Design review of the part built by this model. Coordinates are the model's own, in mm. Face numbers are marked on the shaded views. A direction names the side the tool comes from. Round coordinates to 2 decimals unless told otherwise and drop trailing zeros. Loops run counter-clockwise (first coordinate to the right, second up) from the corner with the lowest first, then second, coordinate; pieces in that order, holes last. Notation, with made-up numbers: M -24.5,34.25 L -17.5,34.25 A7 cw -17.5,46.25 Z; hole C -34.75,-6 d4. An arc over 180 degrees is marked long. Use a Markdown table: item, result.
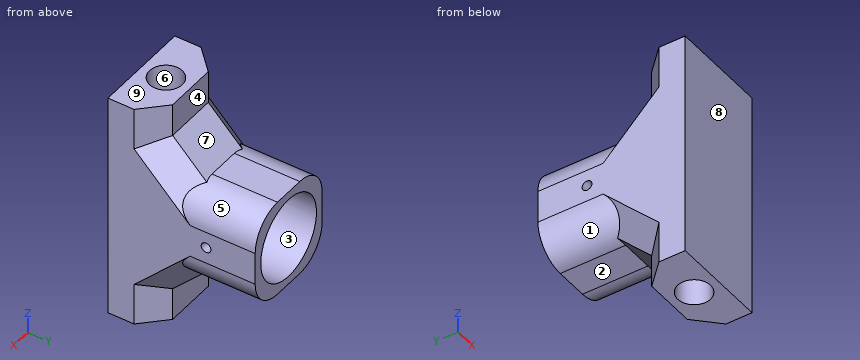
from build123d import *

# Parameters (mm, degrees)
EXTRUDE_1_DEPTH     = 30
SKETCH_2_R          = 12.5
CUT_EXTRUDE_1_DEPTH = 30
SKETCH_3_R          = 5
CUT_EXTRUDE_2_DEPTH = 89.459030065
CHAMFER_1_SIZE      = 10
FILLET_1_R          = 10
CHAMFER_2_SIZE      = 7
SKETCH_4_R          = 1.5
CUT_EXTRUDE_3_DEPTH = 89.459030065


with BuildPart() as part:
    # 草圖1 → 填料-伸長1 (new body)
    with BuildSketch(Plane(origin=(0, 0, 0), x_dir=(0, 0, -1), z_dir=(1, 0, 0))):
        Polygon((50, 15), (70, 15), (70, 0), (0, 0), (0, 15), (20, 15), (20, 45), (50, 45), align=None)
    extrude(amount=EXTRUDE_1_DEPTH)

    # 草圖2 → 除料-伸長1 (cut)
    with BuildSketch(Plane(origin=(0, 45, 0), x_dir=(1, 0, 0), z_dir=(0, 1, 0))):
        with Locations(Location((15, 35, 0), (0, 0, 270))):
            Circle(SKETCH_2_R)
    extrude(amount=-CUT_EXTRUDE_1_DEPTH, mode=Mode.SUBTRACT)

    # 草圖3 → 除料-伸長2 (cut, through all)
    with BuildSketch(Plane.XY):
        with Locations((15, 7.5)):
            Circle(SKETCH_3_R)
    extrude(amount=-CUT_EXTRUDE_2_DEPTH, mode=Mode.SUBTRACT)

    # 導角1
    chamfer_1_edges = [part.edges().sort_by_distance(p)[0] for p in [
        (15, 15, -20),
        (15, 15, -50),
    ]]
    chamfer(chamfer_1_edges, length=CHAMFER_1_SIZE)

    # 圓角1
    fillet_1_edges = [part.edges().sort_by_distance(p)[0] for p in [
        (30, 35, -20),
        (0, 35, -50),
        (30, 35, -50),
        (0, 35, -20),
    ]]
    fillet(fillet_1_edges, radius=FILLET_1_R)

    # 導角2
    chamfer_2_edges = [part.edges().sort_by_distance(p)[0] for p in [
        (0, 15, -5),
        (0, 25, -20),
        (0, 15, -65),
        (0, 25, -50),
        (30, 15, -65),
        (30, 25, -50),
        (30, 15, -5),
        (30, 25, -20),
    ]]
    chamfer(chamfer_2_edges, length=CHAMFER_2_SIZE)

    # 草圖4 → 除料-伸長3 (cut, through all)
    with BuildSketch(Plane(origin=(30, 0, 0), x_dir=(0, 0, -1), z_dir=(1, 0, 0))):
        with Locations((35, 30)):
            Circle(SKETCH_4_R)
    extrude(amount=-CUT_EXTRUDE_3_DEPTH, mode=Mode.SUBTRACT)


solid = part.part
1. Take a section at A-A on z = -35. Give the boundary of the cut face in (x, y), and give its area (3 significant figures).
Check values:
| item | result |
|---|---|
| outline | M 0,0 L 30,0 L 30,28.5 L 27.5,28.5 L 27.5,15 L 2.5,15 L 2.5,28.5 L 0,28.5 Z; M 0,31.5 L 2.5,31.5 L 2.5,45 L 0,45 Z; M 27.5,31.5 L 30,31.5 L 30,45 L 27.5,45 Z; hole C 15,7.5 d10 |
| area | 506 mm² |
2. Take a section at D-D on z = -66. Give the boundary of the cut face in (x, y), and give its area (3 significant figures).
Check values:
| item | result |
|---|---|
| outline | M 0,0 L 30,0 L 30,8 L 23,15 L 7,15 L 0,8 Z; hole C 15,7.5 d10 |
| area | 322 mm² |
3. Wall thickness on line 1 along Y through (x, z) = (28.6, -35); line 2 along Z through (x, y) = (17.5, 34.5); line 3 along Y through (x, z) = (19.5, -28): over which ranges is each line inside the solid? List them lowest first. Write a range as from..to.
Check values:
| item | result |
|---|---|
| line 1 | y = 0..28.5, 31.5..45 |
| line 2 | z = -50..-47.25, -22.75..-20 |
| line 3 | y = 0..5.32, 9.68..15 |
4. Machinability: for the marked faces 1, 2, 3, 4 and 5, which of the approach directions +Z, -Z, +X, -X, +Y, -Y give a long, thin tool a straight path to every point of the face, cutting with its end or side? Answer none if there is none.
Check values:
| item | result |
|---|---|
| face 1 | -Z, -X, +Y |
| face 2 | -Z, +X, -X, +Y |
| face 3 | +Y |
| face 4 | +Z, +X, -X, +Y |
| face 5 | +Z, +X, +Y |
5. Take a section at C-C on x = 15. Give the boundary of the cut face in (y, z), and give its area (3 significant figures).
Check values:
| item | result |
|---|---|
| outline | M 0,-70 L 2.5,-70 L 2.5,0 L 0,0 Z; M 12.5,-70 L 15,-70 L 15,-60 L 25,-50 L 45,-50 L 45,-47.5 L 15,-47.5 L 15,-22.5 L 45,-22.5 L 45,-20 L 25,-20 L 15,-10 L 15,0 L 12.5,0 Z |
| area | 600 mm² |
6. Insertion check: pin 1 (8 mm diameter, centred on y = 26, z = -47, fed in from -X); pin 2 (8 mm diameter, centred on x = 15, y = 34.5, fed in from -Z); pin 3 (5 mm diameter, centred on x = 16.5, z = -6, fed in from +Y); pin 4 (2.5 mm diameter, centred on y = 30, z = -35, fed in from -X). Each pin has a flat end and moves straight along its axis. Give the tip position at first contact, or say it passes through.
Check values:
| item | result |
|---|---|
| pin 1 | stops at x = 0.46 |
| pin 2 | stops at z = -50 |
| pin 3 | stops at y = 15 |
| pin 4 | passes through |
7. The part is to be moulded in two halves that separate along Y. For the marked faces 6, 7, 8 and 9, say which applies: pulls with the +Y half, pulls with the -Y half, needs draft (parallel to the pull), parting line crosses it, or undercut.
Check values:
| item | result |
|---|---|
| face 6 | undercut |
| face 7 | pulls with the +Y half |
| face 8 | pulls with the -Y half |
| face 9 | needs draft |
8. Take a section at B-B on y = 32.5. Give the boundary of the cut face in (x, z).
Check values:
| item | result |
|---|---|
| outline | M 0,-40 A10 ccw 10,-50 L 20,-50 A10 ccw 30,-40 L 30,-30 A10 ccw 20,-20 L 10,-20 A10 ccw 0,-30 Z; hole C 15,-35 d25 |
